CAD build for the part. Positions are in the model's coordinates, mm. A direction names the side the tool comes from. Round coordinates to 2 decimals unless told otherwise and drop trailing zeros. Order: outer loops, then holes, each group sorted by start corner. A loop starts at its lowest first (then second) coordinate and runs counter-clockwise, first axis right, second up. Notation, with made-up numbers: M 1,30 L 19,30 A26 ccw 19,61 Z; hole C 17.5,86.5 d8. An arc over 180 degrees is marked long. Answer as a JSON object with one key per item and string values.
```python
from build123d import *

# Parameters (mm, degrees)
SKETCH1_W                        = 19.05
SKETCH1_H                        = 42.8625
BOSS_EXTRUDE1_DEPTH              = 15.24
F_18_0_1695_DIAMETER_HOLE1_D     = 4.3053
F_18_0_1695_DIAMETER_HOLE1_DEPTH = 15.24
CUT_EXTRUDE1_REACH               = 17.24


with BuildPart() as part:
    # Sketch1 → Boss-Extrude1 (new body)
    with BuildSketch(Plane(origin=(0, 0, 0), x_dir=(1, 0, 0), z_dir=(0, 1, 0))):
        with Locations((-16.213580696, -1.598006412)):
            Rectangle(SKETCH1_W, SKETCH1_H)
    extrude(amount=BOSS_EXTRUDE1_DEPTH)

    # #18 (0.1695) Diameter Hole1
    with Locations(Plane(origin=(0, 15.24, 0), x_dir=(-1, 0, 0), z_dir=(0, 1, 0))):
        with Locations((20.150580696, 17.473006412)):
            Hole(F_18_0_1695_DIAMETER_HOLE1_D / 2, depth=F_18_0_1695_DIAMETER_HOLE1_DEPTH)

    # Sketch4 → Cut-Extrude1 (cut, up to next)
    with BuildSketch(Plane(origin=(0, 15.24, 0), x_dir=(1, 0, 0), z_dir=(0, 1, 0)), mode=Mode.PRIVATE) as cut_extrude1_sk1:
        with BuildLine():
            Line((-17.997930696, 16.004193588), (-17.997930696, 12.549793588))
            ThreePointArc((-17.997930696, 12.549793588), (-20.150580696, 10.397143588), (-22.303230696, 12.549793588))
            Line((-22.303230696, 12.549793588), (-22.303230696, 16.004193588))
            ThreePointArc((-22.303230696, 16.004193588), (-20.150580696, 18.156843588), (-17.997930696, 16.004193588))
        make_face()
    cut_extrude1_tool1 = extrude(cut_extrude1_sk1.sketch, amount=-CUT_EXTRUDE1_REACH, mode=Mode.PRIVATE) & part.part
    add(cut_extrude1_tool1.solids().sort_by_distance((-20.150581, 15.24, -14.276994))[0], mode=Mode.SUBTRACT)


solid = part.part
```
Item 1: 3-axis set-ups, long thin cutter, end or side, ignore diameter. For faces 1 (the flat face through (-16, 8, -19.833)), 2 (the flat face through (-17.998, 8, -14)): which of +Z, -Z, +X, -X, +Y, -Y reach the whole face in a straight line?
Worked answers:
{"face 1": "-Z, +X, -X, +Y, -Y", "face 2": "+Y, -Y"}
Item 2: Two-plate mould, pull along X, no slides. Class faces 3 (the flat face through (-25.739, 8, 2)), 4 (the flat face through (-16, 8, 23.029)), 5 (the cylindrical face through (-19.16, 7.51, 15.56)): released by +X, released by -X, zero draft, split by the parting line, or undercut.
Worked answers:
{"face 3": "released by -X", "face 4": "zero draft", "face 5": "undercut"}
Item 3: Drop flat-ended pins along their axis: pin 1 Ø5 at (x, z) = (-10, 2.5) entering from -Y; pin 2 Ø2.5 at (x, z) = (-20.15, 17.47) entering from +Y. Give the stop position or say it passes through.
Worked answers:
{"pin 1": "stops at y = 0", "pin 2": "passes through"}
Item 4: Saw through at A-A on z = 17. List the corners of the cut face in (x, y), and give its area (3 significant figures).
Worked answers:
{"outline": "M -25.74,0 L -22.25,0 L -22.25,15.24 L -25.74,15.24 Z; M -18.05,0 L -6.69,0 L -6.69,15.24 L -18.05,15.24 Z", "area": "226 mm2"}
Item 5: Wall check: line 1 along X through (y, z) = (11.25, -12.5); line 2 along Z through (x, y) = (-20.25, 1.75); line 3 along Z through (x, y) = (-22, 13.5). Give the ranges that are in metal, low to high. Write a range as [from, to].
Worked answers:
{"line 1": "x = [-25.74, -22.3], [-18, -6.69]", "line 2": "z = [-19.83, -18.15], [-10.4, 15.32], [19.62, 23.03]", "line 3": "z = [-19.83, -17.11], [-11.45, 16.37], [18.57, 23.03]"}
Item 6: Saw through at B-B on y = 4.5. List the corners of the cut face in (x, z), and give its area (3 significant figures).
Worked answers:
{"outline": "M -25.74,-19.83 L -6.69,-19.83 L -6.69,23.03 L -25.74,23.03 Z; hole M -22.3,-16 A2.15 ccw -18,-16 L -18,-12.55 A2.15 ccw -22.3,-12.55 Z; hole C -20.15,17.47 d4.31", "area": "773 mm2"}
